Solid Edge part; units mm, degrees
sketch "Sketch1" plane through (0, 0, 0) normal (0, 0, 1) x (1, 0, 0)
  line L0 (-5.494, 0) -> (-3.8848, -3.8848)
  line L1 (-3.8848, -3.8848) -> (0, -5.494)
  line L2 (0, -5.494) -> (3.8848, -3.8848)
  line L3 (3.8848, -3.8848) -> (5.494, 0)
  line L4 (5.494, 0) -> (3.8848, 3.8848)
  line L5 (3.8848, 3.8848) -> (0, 5.494)
  line L6 (0, 5.494) -> (-3.8848, 3.8848)
  line L7 (-3.8848, 3.8848) -> (-5.494, 0)
extrude "Protrusion1" add sketch "Sketch1" along normal mid plane 3.67
sketch "Sketch2" plane through (0, 0, -1.835) normal (0, 0, -1) x (0.9239, 0.3827, 0)
  circle A0 centre (0, 0) radius 2.675
extrude "ExtrudedProtrusion_2" add sketch "Sketch2" along normal blind 19.07
Work out the finished part from the listing and answer in its coordinate system (mm). Coordinates: 2 decimals unless noted, no trailing zeros. Write each loop counter-clockwise with the first axis right and the second up, starting at its lowest first coordinate (ties: lowest second). Pieces come first, ordered by that corner, then holes. Notation, with made-up numbers: M 27,68 L 32,68 A14 cw 32,74 Z; hole C -29.75,4 d4. An arc over 180 degrees is marked long. Answer as CSV lines item,"result". Start each with the question number.
Item 1: Section A-A on z = 0.25 is taken. Write down the section's boundary in (x, y), and give its area (3 significant figures).
Item 2: Determine the mould class of faces 1 (the face through (4.7, 1.92, -0.03)), 2 (the face through (-4.7, -1.92, -0.03)), 3 (the face through (0.465, 2.634, -11.237)), 4 (the face through (-3, -1, -1.835)) for opening direction X: released by +X, released by -X, zero draft, split by the parting line, or undercut.
Item 3: Section B-B on y = -1 is taken. Write down the section's boundary in (x, z) (3 decimals).
Item 4: Flat-ended cylindrical pins translate along their axes: P1, Ø1.5, axis at y = 1, z = -4, coming from the -X side; P2, Ø5, axis at x = 4, z = -5.5, coming from the -Y side; P3, Ø3, axis at x = -1, z = -10, coming from the +Y side (3 decimals). Find the tip coordinate at first contact, or state that the pin passes through.
Item 5: Section C-C on x = -3.5 is taken. Write down the section's boundary in (y, z) (3 decimals), and give its area (3 significant figures).
Item 6: Section D-D on x = 5.25 is taken. Write down the section's boundary in (y, z) (3 decimals).
Item 7: Consider L1, parallel to Z at x = -3.5, y = 1.25 (3 decimals); L2, parallel to X at y = 0, z = -17 (3 decimals); L3, parallel to Y at x = 4, z = -1.5. Determine where each line is inside the solid, lowest interval first.
Checks:
1,outline,"M -5.49,0 L -3.88,-3.88 L 0,-5.49 L 3.88,-3.88 L 5.49,0 L 3.88,3.88 L 0,5.49 L -3.88,3.88 Z"
1,area,"85.4 mm²"
2,face 1,"released by +X"
2,face 2,"released by -X"
2,face 3,"split by the parting line"
2,face 4,"zero draft"
3,outline,"M -5.08,-1.835 L -2.481,-1.835 L -2.481,-20.905 L 2.481,-20.905 L 2.481,-1.835 L 5.08,-1.835 L 5.08,1.835 L -5.08,1.835 Z"
4,P1,"stops at x = -2.66"
4,P2,"stops at y = -2.21"
4,P3,"stops at y = 2.675"
5,outline,"M -4.044,-1.835 L 4.044,-1.835 L 4.044,1.835 L -4.044,1.835 Z"
5,area,"29.7 mm²"
6,outline,"M -0.589,-1.835 L 0.589,-1.835 L 0.589,1.835 L -0.589,1.835 Z"
7,L1,"z = -1.835 to 1.835"
7,L2,"x = -2.675 to 2.675"
7,L3,"y = -3.61 to 3.61"
